Check sheet for the modelled part. Datum: model origin and axes. Units: mm. A direction names the side the tool comes from. Round coordinates to 2 decimals unless told otherwise and drop trailing zeros. Order: outer loops, then holes, each group sorted by start corner. A loop starts at its lowest first (then second) coordinate and runs counter-clockwise, first axis right, second up. Notation, with made-up numbers: M 59.5,25.5 L 118.5,25.5 A12 cw 118.5,41.5 Z; hole C 22,-16.5 d7. An arc over 180 degrees is marked long. One line per item, written item: value. Start each with the question number.
(1) Cross-section at B-B, the plane z = -177. Enter the section's corners in (x, y).
(2) Cross-section at A-A, the plane x = 198. Enter the section's corners in (y, z), and give its area (3 significant figures).
(3) Depth check by flat-ended pin: pin 1 Ø3 at (x, z) = (317.5, -95.25) entering from +Y; pin 2 Ø3 at (x, z) = (190, -142) entering from -Y; pin 3 Ø1.5 at (x, z) = (12.7, -95.25) entering from +Y; pin 4 Ø4.5 at (x, z) = (316.5, -95) entering from +Y. Enter the tip coordinate at first touch or a pass-through.
(4) Cross-section at C-C, the plane y = 4. Enter the section's corners in (x, z), and give its area (3 significant figures).
(5) Thickness scan on L1, parallel to X at y = 26.5, z = -95.25; L2, parallel to X at y = 50, z = -95; L3, parallel to X at y = 4.5, z = -74. Record the ranges inside material, lowest first.
(6) Release check for a two-part mould opening along X. For faces 1 (the face through (163, 12.7, -100)), 2 (the face through (163, 50.8, -103)), 3 (the face through (330.2, 25, -100)), 4 (the face through (0, 25, -100)) record: released by +X, released by -X, zero draft, split by the parting line, or undercut.
(7) Access from +Z, -Z, +X, -X, +Y, -Y to the whole of each face (thin tool, end or side, straight path). Record for faces 5 (the face through (163, 0, -13)), 6 (the face through (167, 6, -21.934)).
from build123d import *

# Parameters (mm, degrees)
SKETCH1_W                                   = 330.2
SKETCH1_H                                   = 203.2
BOSS_EXTRUDE1_DEPTH                         = 50.8
CUT_EXTRUDE1_DEPTH                          = 12.7
CBORE_FOR_2_BINDING_HEAD_MACHINE_SC_2_COUNT = 2
CBORE_FOR_2_BINDING_HEAD_MACHINE_SC_2_PITCH = 304.799059425


with BuildPart() as part:
    # Sketch1 → Boss-Extrude1 (new body)
    with BuildSketch(Plane(origin=(0, 0, 0), x_dir=(1, 0, 0), z_dir=(0, 1, 0))):
        with Locations((165.1, 101.6)):
            Rectangle(SKETCH1_W, SKETCH1_H)
    extrude(amount=BOSS_EXTRUDE1_DEPTH)

    # Sketch3 → Cut-Extrude1 (cut)
    with BuildSketch(Plane.XZ):
        Polygon((279.4, -181.265982614), (279.4, -104.941398829), (279.4, -104.237946444), (279.4, -21.934017386), (50.8, -21.934017386), (50.8, -181.265982614), align=None)
    extrude(amount=-CUT_EXTRUDE1_DEPTH, mode=Mode.SUBTRACT)

    # Sketch5 → CBORE for #2 Binding Head Machine Screw1 (revolve, cut)
    with BuildSketch(Plane(origin=(12.700940575, 50.8, -95.25), x_dir=(0, 0, 1), z_dir=(1, 0, 0))):
        Polygon((0, 0), (0, 50.8), (1.2192, 50.8), (1.2192, 1.27), (2.77876, 1.27), (2.77876, 0.635), (3.41376, 0), align=None)
    cbore_for_2_binding_head_machine_screw1 = revolve(axis=Axis((12.700940575, 57.15, -95.25), (0, -1, 0)), mode=Mode.SUBTRACT)

    # CBORE for _2 Binding Head Machine Sc 2: CBORE for #2 Binding Head Machine Screw1 ×2
    with Locations(*[(i * CBORE_FOR_2_BINDING_HEAD_MACHINE_SC_2_PITCH, 0, 0) for i in range(1, CBORE_FOR_2_BINDING_HEAD_MACHINE_SC_2_COUNT)]):
        add(cbore_for_2_binding_head_machine_screw1, mode=Mode.SUBTRACT)


solid = part.part
Values found:
1. outline: M 0,0 L 50.8,0 L 50.8,12.7 L 279.4,12.7 L 279.4,0 L 330.2,0 L 330.2,50.8 L 0,50.8 Z
2. outline: M 0,-203.2 L 50.8,-203.2 L 50.8,0 L 0,0 L 0,-21.93 L 12.7,-21.93 L 12.7,-181.27 L 0,-181.27 Z
2. area: 8,300 mm^2
3. pin 1: y = 49.53
3. pin 2: y = 12.7
3. pin 3: through
3. pin 4: y = 50.67
4. outline: M 0,-203.2 L 330.2,-203.2 L 330.2,0 L 0,0 Z; hole C 12.7,-95.25 d2.44; hole M 50.8,-181.27 L 279.4,-181.27 L 279.4,-21.93 L 50.8,-21.93 Z; hole C 317.5,-95.25 d2.44
4. area: 30,700 mm^2
5. L1: 0 to 11.48, 13.92 to 316.28, 318.72 to 330.2
5. L2: 0 to 9.93, 15.47 to 314.73, 320.27 to 330.2
5. L3: 0 to 50.8, 279.4 to 330.2
6. face 1: undercut
6. face 2: zero draft
6. face 3: released by +X
6. face 4: released by -X
7. face 5: +Z, -Z, +X, -X, -Y
7. face 6: -Y
